For this review, take the finished solid that the model builds, in its own axes (mm). A direction names the side the tool comes from. Give positions to 0.01 mm unless a question says otherwise; leave off trailing zeros. Loops run counter-clockwise (first coordinate to the right, second up) from the corner with the lowest first, then second, coordinate; pieces in that order, holes last. Notation, with made-up numbers: M -25,-29 L -19,-29 A21 cw -19,-24 Z; hole C 79,87.5 d7. An arc over 180 degrees is marked long. Use CSV: the item, a comma, the result in double quotes. Start each with the question number.
1. Take a section at A-A, the plane z = 48.5. Write out the cut boundary in (x, y) (3 decimals), and give its area (3 significant figures).
2. Insertion check: P1, Ø6.5, axis at x = -39.28, z = 56.86, coming from the +Y side; P2, Ø5.5, axis at y = 32, z = 32.5, coming from the +X side; P3, Ø12.5, axis at y = 29, z = 59.5, coming from the -X side; P4, Ø9, axis at x = -25.5, z = 31, coming from the +Y side. Each pin has a flat end and moves straight along its axis. Give the tip position at first contact, or say it passes through.
3. Take a section at C-C, the plane z = 30.5. State how many separate pieces and enclosed holes the cut face has, and give its area (3 significant figures).
4. To check wall thickness, follow line 1 (X direction, y = 10.5, z = 28); line 2 (X direction, y = 21, z = 60); line 3 (X direction, y = 37.5, z = 57.5). State the ranges of each line that lie inside material, in increasing order. Write a range as [from, to].
5. Take a section at B-B, the plane y = 23. Write out the cut boundary in (x, z), and give its area (3 significant figures).
6. The part is to be moulded in two halves that separate along X. For faces 3 (the face through (-18.449, 32, 31)), 4 (the face through (-8.289, 32, 44)), 5 (the face through (-61, 19.05, 44)), say which applies: pulls with the +X half, pulls with the -X half, needs draft (parallel to the pull), parting line crosses it, or undercut.
7. Tool access review of faces 1 (the face through (-77.123, 9, 44)), 2 (the face through (-26, 19.05, 29)): name each direction out of +Z, -Z, +X, -X, +Y, -Y from which nothing blocks a thin tool from reaching the whole face with its end or side.
8. Take a section at D-D, the plane x = -46. Write out the cut boundary in (y, z).
from build123d import *

# Parameters (mm, degrees)
SKETCH3_W               = 101.6
SKETCH3_H               = 38.1
BOSS_EXTRUDE2_DEPTH     = 19.05
BOSS_EXTRUDE4_START     = 24.868285686
BOSS_EXTRUDE4_OUTLINE_W = 36.068
BOSS_EXTRUDE4_OUTLINE_H = 25.4
BOSS_EXTRUDE4_DEPTH     = 38.1
CUT_EXTRUDE2_REACH      = 111.036
SKETCH7_R               = 11.049
SKETCH7_R_2             = 1.9812
SKETCH8_W               = 15.748
SKETCH8_H               = 38.1
CUT_EXTRUDE3_DEPTH      = 25.4
CUT_EXTRUDE4_REACH      = 111.036
SKETCH9_R               = 3.302
CUT_EXTRUDE5_REACH      = 98.827
SKETCH11_R              = 3.429


# Read off the part's stored shape, not the designer's step: Boss-Extrude4
with BuildPart() as part:
    # Sketch3 → Boss-Extrude2 (new body)
    with BuildSketch(Plane(origin=(0, 0, 0), x_dir=(1, 0, 0), z_dir=(0, 1, 0))):
        with Locations((-26.323326811, -43.918285686)):
            Rectangle(SKETCH3_W, SKETCH3_H)
    extrude(amount=BOSS_EXTRUDE2_DEPTH)

    # Boss-Extrude4 outline → Boss-Extrude4 (add)
    with BuildSketch(Plane.XY.offset(BOSS_EXTRUDE4_START)):
        with Locations((-26.323326811, 31.75)):
            Rectangle(BOSS_EXTRUDE4_OUTLINE_W, BOSS_EXTRUDE4_OUTLINE_H)
    extrude(amount=BOSS_EXTRUDE4_DEPTH)

    # Sketch7 → Cut-Extrude2 (cut, up to next)
    with BuildSketch(Plane(origin=(0, 44.45, 0), x_dir=(1, 0, 0), z_dir=(0, 1, 0)), mode=Mode.PRIVATE) as cut_extrude2_sk1:
        with Locations(Location((-26.323326811, -43.918285686, 0), (0, 0, 270))):
            Circle(SKETCH7_R)
    cut_extrude2_tool1 = extrude(cut_extrude2_sk1.sketch, amount=-CUT_EXTRUDE2_REACH, mode=Mode.PRIVATE) & part.part
    # Sketch7 → Cut-Extrude2 (cut, up to next)
    with BuildSketch(Plane(origin=(0, 44.45, 0), x_dir=(1, 0, 0), z_dir=(0, 1, 0)), mode=Mode.PRIVATE) as cut_extrude2_sk2:
        with Locations(Location((-13.369326811, -56.863342795, 0), (0, 0, 270))):
            Circle(SKETCH7_R_2)
    cut_extrude2_tool2 = extrude(cut_extrude2_sk2.sketch, amount=-CUT_EXTRUDE2_REACH, mode=Mode.PRIVATE) & part.part
    # Sketch7 → Cut-Extrude2 (cut, up to next)
    with BuildSketch(Plane(origin=(0, 44.45, 0), x_dir=(1, 0, 0), z_dir=(0, 1, 0)), mode=Mode.PRIVATE) as cut_extrude2_sk3:
        with Locations(Location((-39.277326811, -56.863342795, 0), (0, 0, 270))):
            Circle(SKETCH7_R_2)
    cut_extrude2_tool3 = extrude(cut_extrude2_sk3.sketch, amount=-CUT_EXTRUDE2_REACH, mode=Mode.PRIVATE) & part.part
    # Sketch7 → Cut-Extrude2 (cut, up to next)
    with BuildSketch(Plane(origin=(0, 44.45, 0), x_dir=(1, 0, 0), z_dir=(0, 1, 0)), mode=Mode.PRIVATE) as cut_extrude2_sk4:
        with Locations(Location((-39.277326811, -30.955342795, 0), (0, 0, 270))):
            Circle(SKETCH7_R_2)
    cut_extrude2_tool4 = extrude(cut_extrude2_sk4.sketch, amount=-CUT_EXTRUDE2_REACH, mode=Mode.PRIVATE) & part.part
    # Sketch7 → Cut-Extrude2 (cut, up to next)
    with BuildSketch(Plane(origin=(0, 44.45, 0), x_dir=(1, 0, 0), z_dir=(0, 1, 0)), mode=Mode.PRIVATE) as cut_extrude2_sk5:
        with Locations(Location((-13.369326811, -30.955342795, 0), (0, 0, 270))):
            Circle(SKETCH7_R_2)
    cut_extrude2_tool5 = extrude(cut_extrude2_sk5.sketch, amount=-CUT_EXTRUDE2_REACH, mode=Mode.PRIVATE) & part.part
    add(cut_extrude2_tool1.solids().sort_by_distance((-26.323327, 44.45, 43.918286))[0], mode=Mode.SUBTRACT)
    add(cut_extrude2_tool2.solids().sort_by_distance((-13.369327, 44.45, 56.863343))[0], mode=Mode.SUBTRACT)
    add(cut_extrude2_tool3.solids().sort_by_distance((-39.277327, 44.45, 56.863343))[0], mode=Mode.SUBTRACT)
    add(cut_extrude2_tool4.solids().sort_by_distance((-39.277327, 44.45, 30.955343))[0], mode=Mode.SUBTRACT)
    add(cut_extrude2_tool5.solids().sort_by_distance((-13.369327, 44.45, 30.955343))[0], mode=Mode.SUBTRACT)

    # Sketch8 → Cut-Extrude3 (cut)
    with BuildSketch(Plane(origin=(0, 44.45, 0), x_dir=(1, 0, 0), z_dir=(0, 1, 0))):
        with Locations((-26.323326811, -43.918285686)):
            Rectangle(SKETCH8_W, SKETCH8_H)
    extrude(amount=-CUT_EXTRUDE3_DEPTH, mode=Mode.SUBTRACT)

    # Sketch9 → Cut-Extrude4 (cut, up to next)
    with BuildSketch(Plane.XZ, mode=Mode.PRIVATE) as cut_extrude4_sk1:
        with Locations(Location((14.316673189, 52.808285686, 0), (0, 0, 270))):
            Circle(SKETCH9_R)
    cut_extrude4_tool1 = extrude(cut_extrude4_sk1.sketch, amount=-CUT_EXTRUDE4_REACH, mode=Mode.PRIVATE) & part.part
    # Sketch9 → Cut-Extrude4 (cut, up to next)
    with BuildSketch(Plane.XZ, mode=Mode.PRIVATE) as cut_extrude4_sk2:
        with Locations(Location((-66.963326811, 52.808285686, 0), (0, 0, 270))):
            Circle(SKETCH9_R)
    cut_extrude4_tool2 = extrude(cut_extrude4_sk2.sketch, amount=-CUT_EXTRUDE4_REACH, mode=Mode.PRIVATE) & part.part
    add(cut_extrude4_tool1.solids().sort_by_distance((14.316673, 0, 52.808286))[0], mode=Mode.SUBTRACT)
    add(cut_extrude4_tool2.solids().sort_by_distance((-66.963327, 0, 52.808286))[0], mode=Mode.SUBTRACT)

    # Sketch11 → Cut-Extrude5 (cut, up to next)
    with BuildSketch(Plane(origin=(0, 0, 24.868285686), x_dir=(-1, 0, 0), z_dir=(0, 0, -1)), mode=Mode.PRIVATE) as cut_extrude5_sk1:
        with Locations((7.527326811, 9.525)):
            Circle(SKETCH11_R)
    cut_extrude5_tool1 = extrude(cut_extrude5_sk1.sketch, amount=-CUT_EXTRUDE5_REACH, mode=Mode.PRIVATE) & part.part
    # Sketch11 → Cut-Extrude5 (cut, up to next)
    with BuildSketch(Plane(origin=(0, 0, 24.868285686), x_dir=(-1, 0, 0), z_dir=(0, 0, -1)), mode=Mode.PRIVATE) as cut_extrude5_sk2:
        with Locations((45.119326811, 9.525)):
            Circle(SKETCH11_R)
    cut_extrude5_tool2 = extrude(cut_extrude5_sk2.sketch, amount=-CUT_EXTRUDE5_REACH, mode=Mode.PRIVATE) & part.part
    add(cut_extrude5_tool1.solids().sort_by_distance((-7.527327, 9.525, 24.868286))[0], mode=Mode.SUBTRACT)
    add(cut_extrude5_tool2.solids().sort_by_distance((-45.119327, 9.525, 24.868286))[0], mode=Mode.SUBTRACT)


solid = part.part
Result set:
1,outline,"M -77.123,0 L -36.378,0 L -36.378,44.45 L -44.357,44.45 L -44.357,19.05 L -77.123,19.05 Z; M -16.269,0 L 24.477,0 L 24.477,19.05 L -8.289,19.05 L -8.289,44.45 L -16.269,44.45 Z; hole C -45.119,9.525 d6.858; hole C -7.527,9.525 d6.858"
1,area,"1,880 mm2"
2,P1,"y = 44.45"
2,P2,"x = -8.29"
2,P3,"x = -44.36"
2,P4,"y = 19.05"
3,separate pieces,"3"
3,enclosed holes,"2"
3,area,"2,030 mm2"
4,line 1,"[-77.12, -48.41], [-41.83, -10.81], [-4.24, 24.48]"
4,line 2,"[-44.36, -34.2], [-18.45, -8.29]"
4,line 3,"[-44.36, -41.15], [-37.4, -34.2], [-18.45, -15.25], [-11.49, -8.29]"
5,outline,"M -44.36,24.87 L -34.2,24.87 L -34.2,36.17 A11.05 cw -34.2,51.67 L -34.2,62.97 L -44.36,62.97 Z; M -18.45,24.87 L -8.29,24.87 L -8.29,62.97 L -18.45,62.97 L -18.45,51.67 A11.05 cw -18.45,36.17 Z; hole C -39.28,30.96 d3.96; hole C -39.28,56.86 d3.96; hole C -13.37,30.96 d3.96; hole C -13.37,56.86 d3.96"
5,area,"657 mm2"
6,face 3,"undercut"
6,face 4,"pulls with the +X half"
6,face 5,"needs draft"
7,face 1,"+Z, -Z, -X, +Y, -Y"
7,face 2,"+Z, -Z, +Y"
8,outline,"M 0,24.87 L 6.21,24.87 L 6.21,62.97 L 0,62.97 Z; M 12.84,24.87 L 19.05,24.87 L 19.05,62.97 L 12.84,62.97 Z"
